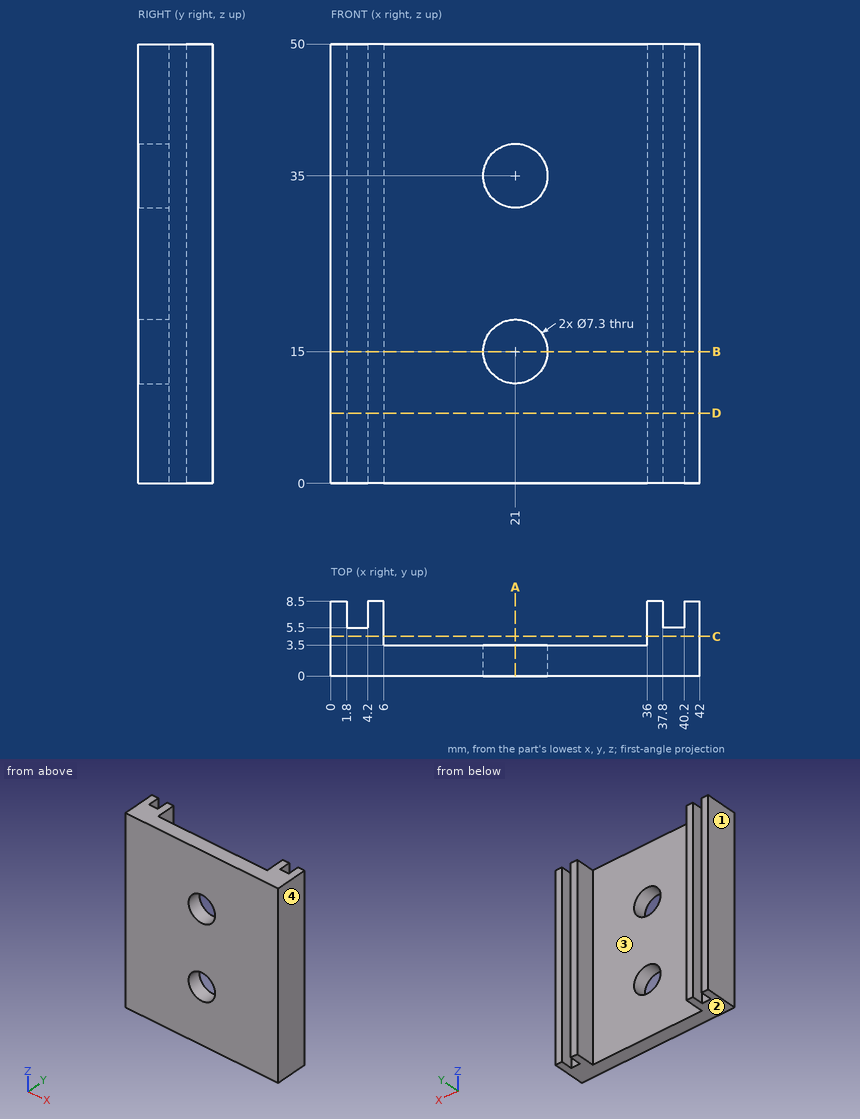
Job drawing, mm, ordinate dimensions from the low corner. One solid piece. Give positions to 0.01 mm unless a question says otherwise; leave off trailing zeros. Loops run counter-clockwise (first coordinate to the right, second up) from the corner with the lowest first, then second, coordinate; pieces in that order, holes last. Notation, with made-up numbers: (77.25, -23) -> (123.25, -23) arc R17 ccw to (123.25, -5) -> close; hole circle Ø2 at (84, 5.25). An arc over 180 degrees is marked (long way). Write each question's results on one line, items separated by ' | '.
(1) Probe line 1 along Z through (x, y) = (21, 1.55); line 2 along X through (y, z) = (8, 29.5); line 3 along X through (y, z) = (4.5, 13.5). List the from-to ranges inside material, lowest first.
Geometry results:
line 1: z = 0 to 11.35, 18.65 to 31.35, 38.65 to 50 | line 2: x = 0 to 1.8, 4.2 to 6, 36 to 37.8, 40.2 to 42 | line 3: x = 0 to 6, 36 to 42
(2) Cut at D-D on z = 8. List the corners of the cut face in (x, y).
Geometry results:
outline: (0, 0) -> (42, 0) -> (42, 8.5) -> (40.2, 8.5) -> (40.2, 5.5) -> (37.8, 5.5) -> (37.8, 8.5) -> (36, 8.5) -> (36, 3.5) -> (6, 3.5) -> (6, 8.5) -> (4.2, 8.5) -> (4.2, 5.5) -> (1.8, 5.5) -> (1.8, 8.5) -> (0, 8.5) -> close
(3) Pull direction X, two halves, no side cores. Call the marked faces 1, 2, 3 and 4: released by +X, released by -X, zero draft, split by the parting line, or undercut.
Geometry results:
face 1: released by -X | face 2: zero draft | face 3: undercut | face 4: released by +X
(4) Flat gauge pins, fed straight in: pin 1 Ø2.5 at (y, z) = (7.5, 14) entering from -X; pin 2 Ø0.7 at (x, z) = (39.5, 26.5) entering from +Y; pin 3 Ø15 at (x, z) = (14.5, 13.5) entering from +Y. Where does each tip first touch, or does it go through?
Geometry results:
pin 1: stops at x = 0 | pin 2: stops at y = 5.5 | pin 3: stops at y = 3.5
(5) Cut at B-B on z = 15. List the corners of the cut face in (x, y).
Geometry results:
outline: (0, 0) -> (17.35, 0) -> (17.35, 3.5) -> (6, 3.5) -> (6, 8.5) -> (4.2, 8.5) -> (4.2, 5.5) -> (1.8, 5.5) -> (1.8, 8.5) -> (0, 8.5) -> close; (24.65, 0) -> (42, 0) -> (42, 8.5) -> (40.2, 8.5) -> (40.2, 5.5) -> (37.8, 5.5) -> (37.8, 8.5) -> (36, 8.5) -> (36, 3.5) -> (24.65, 3.5) -> close
(6) Cut at A-A on x = 21. List the corners of the cut face in (y, z), and give its area (3 significant figures).
Geometry results:
outline: (0, 0) -> (3.5, 0) -> (3.5, 11.35) -> (0, 11.35) -> close; (0, 18.65) -> (3.5, 18.65) -> (3.5, 31.35) -> (0, 31.35) -> close; (0, 38.65) -> (3.5, 38.65) -> (3.5, 50) -> (0, 50) -> close | area: 124 mm²
(7) Cut at C-C on y = 4.5. List the corners of the cut face in (x, z).
Geometry results:
outline: (0, 0) -> (6, 0) -> (6, 50) -> (0, 50) -> close; (36, 0) -> (42, 0) -> (42, 50) -> (36, 50) -> close
